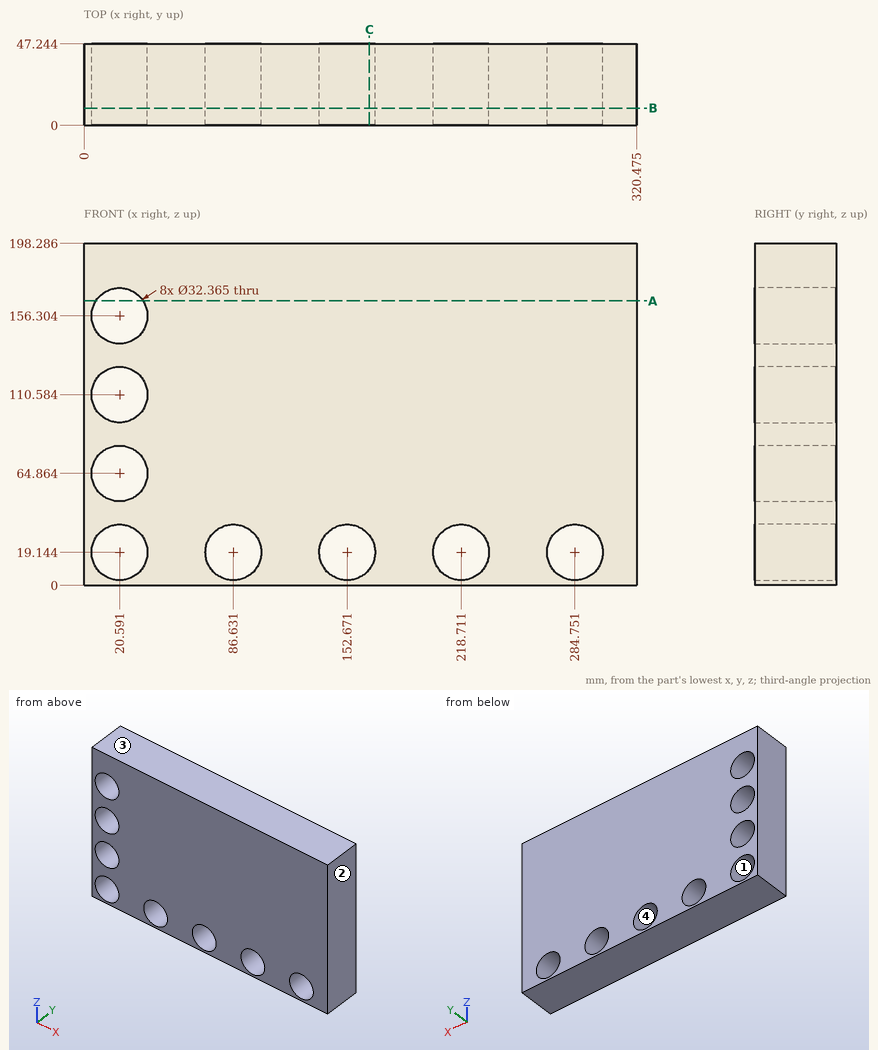
The figure shows three views and two pictorial views of one solid part (mm, origin at its lowest corner). Answer the questions. Round coordinates to 2 decimals unless told otherwise and drop trailing zeros. Write each loop counter-clockwise with the first axis right and the second up, starting at its lowest first coordinate (ties: lowest second). Pieces come first, ordered by that corner, then holes. Notation, with made-up numbers: (-5.5, 31) - (2.5, 31) arc R14 cw to (2.5, 38) - close; hole circle Ø9 at (50.25, 31.25). An arc over 180 degrees is marked (long way). Answer in a Markdown table with one row per item. Add a question column.
1. Find the intervals of material crossed by line 1 along X through (y, z) = (36, 109.5) (1 decimal); line 2 along X through (y, z) = (21, 31.5) (1 decimal); line 3 along Z through (x, y) = (15.5, 26.5) (1 decimal), in increasing order. Write a range as from..to.
2. Given pin 1 (5 mm diameter, centred on x = 134, y = 36.5, fed in from -Z), flat-ended and moving along its own axis, determine where the tip first touches the part or whether it passes through.
3. A cutting plane is placed at B-B, the plane y = 10. Count the separate pieces of the cut face and the enclosed holes in it, and give its area (3 significant figures).
4. A cutting plane is placed at A-A, the plane z = 165. Determine the outline of the cut face in (x, y) (1 decimal).
5. A cutting plane is placed at C-C, the plane x = 165.5. Determine the outline of the cut face in (y, z) (1 decimal).
6. The mould has two halves that part along Z. Classify the marked faces 1, 2, 3 and 4: +Z half, -Z half, draft (parallel to the pull), parting line (faces both ways), or undercut.
Worked out:
| question | item | result |
|---|---|---|
| 1 | line 1 | 0..4.4, 36.7..320.5 |
| 1 | line 2 | 0..10.1, 31..76.2, 97.1..142.2, 163.1..208.3, 229.2..274.3, 295.2..320.5 |
| 1 | line 3 | 0..3.8, 34.5..49.5, 80.2..95.2, 125.9..140.9, 171.7..198.3 |
| 2 | pin 1 | z = 0 |
| 3 | separate pieces | 1 |
| 3 | enclosed holes | 8 |
| 3 | area | 57,000 mm^2 |
| 4 | outline | (0, 0) - (6.9, 0) - (6.9, 47.2) - (0, 47.2) - close; (34.2, 0) - (320.5, 0) - (320.5, 47.2) - (34.2, 47.2) - close |
| 5 | outline | (0, 0) - (47.2, 0) - (47.2, 9.3) - (0, 9.3) - close; (0, 29) - (47.2, 29) - (47.2, 198.3) - (0, 198.3) - close |
| 6 | face 1 | undercut |
| 6 | face 2 | draft |
| 6 | face 3 | +Z half |
| 6 | face 4 | undercut |
